Geometry: final body of the model. Coordinates: model frame, mm. A direction names the side the tool comes from. Coordinates: 2 decimals unless noted, no trailing zeros. Loops run counter-clockwise (first coordinate to the right, second up) from the corner with the lowest first, then second, coordinate; pieces in that order, holes last. Notation, with made-up numbers: M 16.5,73 L 52.5,73 A35 cw 52.5,106 Z; hole C -23,72 d8. An arc over 180 degrees is marked long. Write item = value, one per line. Start each with the question number.
```python
from build123d import *

# Parameters (mm, degrees)
SKETCH4_R            = 72.5
BOSS_EXTRUDE7_DEPTH  = 25
SKETCH13_R           = 72.5
BOSS_EXTRUDE8_DEPTH  = 5
SKETCH14_R           = 20
CUT_EXTRUDE1_DEPTH   = 25
SKETCH15_R           = 20
SKETCH15_R_2         = 10
BOSS_EXTRUDE10_DEPTH = 20


with BuildPart() as part:
    # Sweep1: sweep along a path in Sketch1
    with BuildLine(Plane(origin=(0, 0, 0), x_dir=(0, 0, -1), z_dir=(1, 0, 0))) as sweep1_path:
        CenterArc((0, 0), 72.5, 0, 360)
    # Sketch3 → Sweep1 (sweep)
    with BuildSketch(Plane.XY):
        with BuildLine():
            Line((10, 72.5), (10, 62.5))
            Line((10, 62.5), (-10, 62.5))
            Line((-10, 62.5), (-10, 72.5))
            ThreePointArc((-10, 72.5), (0, 82.5), (10, 72.5))
        make_face()
    sweep(path=sweep1_path.line)



with BuildPart() as body_2:
    # Sketch4 → Boss-Extrude7 (new body, symmetric)
    with BuildSketch(Plane(origin=(0, 0, 0), x_dir=(0, 0, -1), z_dir=(1, 0, 0))):
        Circle(SKETCH4_R)
        with BuildLine():
            Line((25, 0), (62.5, 0))
            ThreePointArc((62.5, 0), (59.441032268, 19.313562148), (50.563562148, 36.736578268))
            Line((50.563562148, 36.736578268), (20.225424859, 14.694631307))
            ThreePointArc((20.225424859, 14.694631307), (23.776412907, 7.725424859), (25, 0))
        make_face(mode=Mode.SUBTRACT)
        with BuildLine():
            Line((7.725424859, 23.776412907), (19.313562148, 59.441032268))
            ThreePointArc((19.313562148, 59.441032268), (0, 62.5), (-19.313562148, 59.441032268))
            Line((-19.313562148, 59.441032268), (-7.725424859, 23.776412907))
            ThreePointArc((-7.725424859, 23.776412907), (0, 25), (7.725424859, 23.776412907))
        make_face(mode=Mode.SUBTRACT)
        with BuildLine():
            Line((7.725424859, -23.776412907), (19.313562148, -59.441032268))
            ThreePointArc((19.313562148, -59.441032268), (36.736578268, -50.563562148), (50.563562148, -36.736578268))
            Line((50.563562148, -36.736578268), (20.225424859, -14.694631307))
            ThreePointArc((20.225424859, -14.694631307), (14.694631307, -20.225424859), (7.725424859, -23.776412907))
        make_face(mode=Mode.SUBTRACT)
        with BuildLine():
            Line((-20.225424859, -14.694631307), (-50.563562148, -36.736578268))
            ThreePointArc((-50.563562148, -36.736578268), (-36.736578268, -50.563562148), (-19.313562148, -59.441032268))
            Line((-19.313562148, -59.441032268), (-7.725424859, -23.776412907))
            ThreePointArc((-7.725424859, -23.776412907), (-14.694631307, -20.225424859), (-20.225424859, -14.694631307))
        make_face(mode=Mode.SUBTRACT)
        with BuildLine():
            Line((-20.225424859, 14.694631307), (-50.563562148, 36.736578268))
            ThreePointArc((-50.563562148, 36.736578268), (-59.441032268, 19.313562148), (-62.5, 0))
            Line((-62.5, 0), (-25, 0))
            ThreePointArc((-25, 0), (-23.776412907, 7.725424859), (-20.225424859, 14.694631307))
        make_face(mode=Mode.SUBTRACT)
    extrude(amount=BOSS_EXTRUDE7_DEPTH, both=True)

    # Sketch12 → Cut-Revolve11 (revolve, cut)
    with BuildSketch(Plane.XY):
        Polygon((-25, 0), (-32.140648249, 0), (-32.140648249, 73.19155482), (-5.016609541, 73.19155482), align=None)
        Polygon((25, 0), (32.140648249, 0), (32.140648249, 73.19155482), (5.016609541, 73.19155482), align=None)
    revolve(axis=Axis((-46.840153715, 0, 0), (1, 0, 0)), mode=Mode.SUBTRACT)


with BuildPart() as part_1:
    add(part.part)

    add(body_2.part)  # Boss-Extrude8 merges body 2
    # Sketch13 → Boss-Extrude8 (add, symmetric)
    with BuildSketch(Plane(origin=(0, 0, 0), x_dir=(0, 0, -1), z_dir=(1, 0, 0))):
        Circle(SKETCH13_R)
    extrude(amount=BOSS_EXTRUDE8_DEPTH, both=True)

    # Sketch14 → Cut-Extrude1 (cut, symmetric)
    with BuildSketch(Plane(origin=(0, 0, 0), x_dir=(0, 0, -1), z_dir=(1, 0, 0))):
        Circle(SKETCH14_R)
    extrude(amount=CUT_EXTRUDE1_DEPTH, both=True, mode=Mode.SUBTRACT)

    # Sketch15 → Boss-Extrude10 (add, symmetric)
    with BuildSketch(Plane(origin=(0, 0, 0), x_dir=(0, 0, -1), z_dir=(1, 0, 0))):
        Circle(SKETCH15_R)
        Circle(SKETCH15_R_2, mode=Mode.SUBTRACT)
    extrude(amount=BOSS_EXTRUDE10_DEPTH, both=True)


solid = part_1.part
```
Item 1: First-contact query: pin 1 (2 mm diameter, centred on y = -2.5, z = 31.5, fed in from -X); pin 2 (4 mm diameter, centred on x = -4.5, y = 40.5, fed in from +Z); pin 3 (5 mm diameter, centred on y = 47, z = -24, fed in from -X). Flat tips, straight axial feed; report the tip coordinate or a pass-through.
Item 2: Line query: line 1 (Y direction, x = 6.15, z = 0); line 2 (Y direction, x = 6.9, z = 0); line 3 (X direction, y = -62, z = -19). Output: solid intervals per line, ascending. Write a range as from..to.
Item 3: Section query A-A (x = 14). Return the cut outline in (y, z).
Item 4: Section query B-B (x = -15). Return the cut outline in (y, z), plus the area to 3 significant figures.
Item 5: Section query C-C (x = -1). Return the cut outline in (y, z), plus the area to 3 significant figures.
Item 6: Pull-direction query (Y, two-part tool) for faces 4 (the flat face through (5, 15, -41)), 5 (the flat face through (20, 9, 5)), 6 (the cylindrical face through (19.773, 6.007, -19.076)); classes: released by +Y, released by -Y, zero draft, split by the parting line, or undercut.
Item 7: Reachability of faces 1 (the cylindrical face through (11.68, 7.62, 23.81)), 2 (the cylindrical face through (-0.28, -9.76, 2.17)), 3 (the flat face through (-10.03, 37.4, -12.15)) from +Z, -Z, +X, -X, +Y, -Y: full face, straight path, thin tool, end or side. Return the list, or none.
Verdict:
q1.pin_1 = -16.65
q1.pin_2 = 72.12
q1.pin_3 = -11.27
q2.line_1 = -80.39..-10, 10..25, 62.5..80.39
q2.line_2 = -79.74..-10, 10..25, 62.5..79.74
q2.line_3 = -10..10
q3.outline = M -38.32,-12.45 L -23.78,-7.73 A25 ccw -14.69,-20.23 L -23.68,-32.59 A40.29 ccw 0,-40.29 L 0,-25 A25 ccw 14.69,-20.23 L 23.68,-32.59 A40.29 ccw 38.32,-12.45 L 23.78,-7.73 A25 ccw 23.78,7.73 L 38.32,12.45 A40.29 ccw 23.68,32.59 L 14.69,20.23 A25 ccw 0,25 L 0,40.29 A40.29 ccw -23.68,32.59 L -14.69,20.23 A25 ccw -23.78,7.73 L -38.32,12.45 A40.29 ccw Z; hole C 0,0 d20
q4.outline = M -34.83,-11.32 L -23.78,-7.73 A25 ccw -14.69,-20.23 L -21.53,-29.63 A36.63 ccw 0,-36.63 L 0,-25 A25 ccw 14.69,-20.23 L 21.53,-29.63 A36.63 ccw 34.83,-11.32 L 23.78,-7.73 A25 ccw 23.78,7.73 L 34.83,11.32 A36.63 ccw 21.53,29.63 L 14.69,20.23 A25 ccw 0,25 L 0,36.63 A36.63 ccw -21.53,29.63 L -14.69,20.23 A25 ccw -23.78,7.73 L -34.83,11.32 A36.63 ccw Z; hole C 0,0 d20
q4.area = 2,770 mm2
q5.outline = C 0,0 d164.9; hole C 0,0 d20
q5.area = 21,000 mm2
q6.face_4 = undercut
q6.face_5 = zero draft
q6.face_6 = split by the parting line
q7.face_1 = +X
q7.face_2 = +X, -X
q7.face_3 = -X
